from build123d import *

# Parameters (mm, degrees)
F0_W     = 20
F0_H     = 8
F1_DEPTH = 4
F0_H_2   = 2
F2_DEPTH = 8
F3_W     = 20
F3_H     = 2
F4_DEPTH = 0.5
F5_R     = 1


with BuildPart() as f1:
    # F0 (on Front) → F1 (new body)
    with BuildSketch(Plane.XZ):
        with Locations((5, 0)):
            Rectangle(F0_W, F0_H)
    extrude(amount=F1_DEPTH)

    # F0 (on Front) → F2 (join)
    with BuildSketch(Plane.XZ):
        with Locations((5, 5)):
            Rectangle(F0_W, F0_H_2)
        with Locations((5, -5)):
            Rectangle(F0_W, F0_H_2)
    extrude(amount=F2_DEPTH)

    # F3 (on face) → F4 (join)
    with BuildSketch(Plane(origin=(0, 0, 4), x_dir=(1, 0, 0), z_dir=(0, 0, -1))):
        with Locations((5, 7)):
            Rectangle(F3_W, F3_H)
    extrude(amount=F4_DEPTH)

    # F5
    f5_edges = [f1.edges().sort_by_distance(p)[0] for p in [
        (5, -8, 3.5),
        (5, -8, -4),
    ]]
    fillet(f5_edges, radius=F5_R)


solid = f1.part
The listing builds one solid part. Answer for the finished solid, in the listing's coordinates (mm). A direction names the side the tool comes from. Give positions to 0.01 mm unless a question says otherwise; leave off trailing zeros. Loops run counter-clockwise (first coordinate to the right, second up) from the corner with the lowest first, then second, coordinate; pieces in that order, holes last. Notation, with made-up numbers: (67, -29) - (73, -29) arc R26 ccw to (73, 7) - close; hole circle Ø3 at (-38, 25). An arc over 180 degrees is marked (long way). Use one line per item in the form item = value.
1. Section A-A on y = -6.5 is taken. Give the vertices of the cut face in (x, z), then the cut area to 3 significant figures.
Calculated:
outline = (-5, -6) - (15, -6) - (15, -4) - (-5, -4) - close; (-5, 3.5) - (15, 3.5) - (15, 6) - (-5, 6) - close
area = 90.0 mm^2
2. Section C-C on z = 3.75 is taken. Give the vertices of the cut face in (x, y), then the cut area to 3 significant figures.
Calculated:
outline = (-5, -7.66) - (15, -7.66) - (15, -6) - (-5, -6) - close; (-5, -4) - (15, -4) - (15, 0) - (-5, 0) - close
area = 113 mm^2
3. Which of the six approach directions +Z, -Z, +X, -X, +Y, -Y give full straight-line access (tool end or side, diameter ignored) to faces 5 (the face through (4.9, -8, -5.5)), 6 (the face through (5, -5, 4)), 7 (the face through (5.14, -7.715, 3.801))?
Calculated:
face_5 = +Z, -Z, +X, -X, -Y
face_6 = +X, -X
face_7 = +X, -X, -Y
4. Find the intervals of material crossed by line 1 along Z through (x, y) = (-3.5, -6.5); line 2 along Y through (x, z) = (3.75, -2.25); line 3 along Z through (x, y) = (10.5, -4.75), in increasing order. Write a range as [from, to].
Calculated:
line_1 = [-6, -4], [3.5, 6]
line_2 = [-4, 0]
line_3 = [-6, -4], [4, 6]
5. Section B-B on x = -1 is taken. Give the vertices of the cut face in (y, z).
Calculated:
outline = (-8, -6) - (0, -6) - (0, 6) - (-8, 6) - (-8, 4.5) arc R1 ccw to (-7, 3.5) - (-6, 3.5) - (-6, 4) - (-4, 4) - (-4, -4) - (-7, -4) arc R1 ccw to (-8, -5) - close
6. Section D-D on z = -2.25 is taken. Give the vertices of the cut face in (x, y).
Calculated:
outline = (-5, -4) - (15, -4) - (15, 0) - (-5, 0) - close
7. Given pin 1 Ø6.5 at (x, z) = (7, -2) entering from -Y, flat-ended and moving along its own axis, determine where the tip first touches the part or whether it passes through.
Calculated:
pin_1 = -8
8. The mould has two halves that part along Z. Classify faces 1 (the face through (5, -4, 6)), 2 (the face through (5, -8, 5)), 3 (the face through (5.14, -7.699, -4.285)), 4 (the face through (5, -5, -4)): pulls with the +Z half, pulls with the -Z half, needs draft (parallel to the pull), parting line crosses it, or undercut.
Calculated:
face_1 = pulls with the +Z half
face_2 = needs draft
face_3 = undercut
face_4 = undercut
